Design review of the part built by this model. Coordinates are the model's own, in mm. Face numbers are marked on the shaded views. A direction names the side the tool comes from. Give positions to 0.01 mm unless a question says otherwise; leave off trailing zeros. Loops run counter-clockwise (first coordinate to the right, second up) from the corner with the lowest first, then second, coordinate; pieces in that order, holes last. Notation, with made-up numbers: (31.25, -23.75) - (73.25, -23.75) arc R24 ccw to (73.25, -5.75) - close; hole circle Ø10 at (35, -4). An arc over 180 degrees is marked (long way). One line per item, written item: value. Start each with the question number.
```python
from build123d import *

# Parameters (mm, degrees)
SKETCH1_R           = 10.5
BOSS_EXTRUDE2_DEPTH = 2
SKETCH2_W           = 40
SKETCH2_H           = 2
BOSS_EXTRUDE3_DEPTH = 35
CUT_EXTRUDE1_DEPTH  = 35
CIRPATTERN1_COUNT   = 3
SKETCH5_R           = 1.5
CUT_EXTRUDE2_DEPTH  = 35
SKETCH6_R           = 1.5
CUT_EXTRUDE3_DEPTH  = 35


with BuildPart() as part:
    # Sketch1 → Boss-Extrude2 (new body)
    with BuildSketch(Plane(origin=(0, 0, 0), x_dir=(1, 0, 0), z_dir=(0, 1, 0))):
        with BuildLine():
            Line((-18.229166667, 5.4375), (-18.229166667, -21.5625))
            Line((-18.229166667, -21.5625), (21.770833333, -21.5625))
            Line((21.770833333, -21.5625), (21.770833333, 5.4375))
            ThreePointArc((21.770833333, 5.4375), (1.770833333, 25.4375), (-18.229166667, 5.4375))
        make_face()
        with Locations(Location((1.770833333, 5.4375, 0), (0, 0, 270))):
            Circle(SKETCH1_R, mode=Mode.SUBTRACT)
    extrude(amount=BOSS_EXTRUDE2_DEPTH)

    # Sketch2 → Boss-Extrude3 (add)
    with BuildSketch(Plane(origin=(0, 2, 0), x_dir=(1, 0, 0), z_dir=(0, 1, 0))):
        with Locations((1.770833333, -20.5625)):
            Rectangle(SKETCH2_W, SKETCH2_H)
    extrude(amount=BOSS_EXTRUDE3_DEPTH)

    # Sketch4 → Cut-Extrude1 (cut)
    with BuildSketch(Plane(origin=(0, 2, 0), x_dir=(1, 0, 0), z_dir=(0, 1, 0))):
        with BuildLine():
            ThreePointArc((1.770833333, 21.4375), (0.770833333, 20.4375), (1.770833333, 19.4375))
            Line((1.770833333, 19.4375), (1.770833333, 21.4375))
        make_face()
        with BuildLine():
            Line((1.770833333, 21.4375), (1.770833333, 19.4375))
            ThreePointArc((1.770833333, 19.4375), (2.477940115, 19.730393219), (2.770833333, 20.4375))
            ThreePointArc((2.770833333, 20.4375), (2.477940115, 21.144606781), (1.770833333, 21.4375))
        make_face()
    cut_extrude1 = extrude(amount=-CUT_EXTRUDE1_DEPTH, mode=Mode.SUBTRACT)

    # CirPattern1: Cut-Extrude1 ×3 about axis
    cirpattern1_axis = Axis((1.770833333, 0, -5.4375), (0, 1, 0))
    for i in range(1, CIRPATTERN1_COUNT):
        add(cut_extrude1.rotate(cirpattern1_axis, i * 360 / CIRPATTERN1_COUNT), mode=Mode.SUBTRACT)

    # Sketch5 → Cut-Extrude2 (cut)
    with BuildSketch(Plane(origin=(0, 0, 19.5625), x_dir=(-1, 0, 0), z_dir=(0, 0, -1))):
        with Locations((-16.466888349, 10.262371912)):
            Circle(SKETCH5_R)
        with Locations((-16.470833333, 30.952470071)):
            Circle(SKETCH5_R)
    extrude(amount=-CUT_EXTRUDE2_DEPTH, mode=Mode.SUBTRACT)

    # Sketch6 → Cut-Extrude3 (cut)
    with BuildSketch(Plane(origin=(0, 0, 19.5625), x_dir=(-1, 0, 0), z_dir=(0, 0, -1))):
        with Locations((12.929166667, 30.96416702)):
            Circle(SKETCH6_R)
        with Locations((12.929166667, 10.470851603)):
            Circle(SKETCH6_R)
    extrude(amount=-CUT_EXTRUDE3_DEPTH, mode=Mode.SUBTRACT)


solid = part.part
```
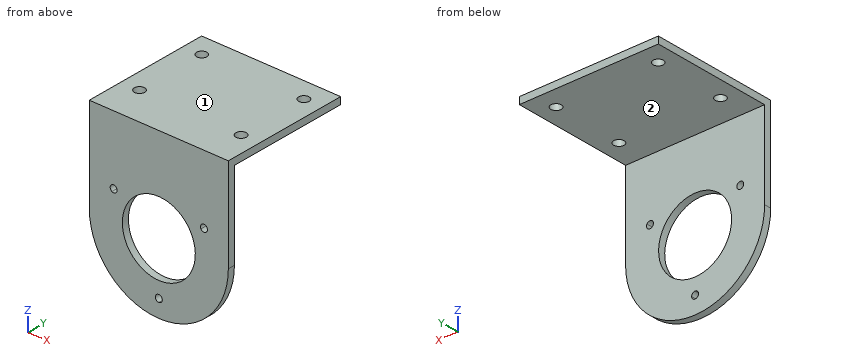
(1) Take a section at D-D on y = 19. State the section outline as (x, z) points.
(2) Take a section at B-B on z = -4. State the section outline as (x, y) points, and give its area (3 significant figures).
(3) For pin 1 Ø10.5 at (x, y) = (0, 21) entering from -Z; pin 2 Ø1.5 at (x, z) = (-11, 3.5) entering from +Y, all flat-tipped, find the tip position at first contact; note any pin that passes through.
(4) To check wall thickness, follow L1, parallel to Y at x = 1.5, z = 11.5; L2, parallel to Z at x = -3, y = 32. State the ranges of each line that lie inside material, in increasing order. Write a range as from..to.
(5) Machinability: for the marked faces 1 and 2, which of the approach directions +Z, -Z, +X, -X, +Y, -Y give a long, thin tool a straight path to every point of the face, cutting with its end or side? Answer none if there is none.
(6) Take a section at A-A on x = 7. State the section outline as (y, z) points.
(7) Take a section at C-C on z = 12. State the section outline as (x, y) points, and give its area (3 significant figures).
Here are the results:
1. outline: (-18.23, 19.56) - (21.77, 19.56) - (21.77, 21.56) - (-18.23, 21.56) - close
2. outline: (-18.23, 0) - (-8.63, 0) - (-8.63, 2) - (-18.23, 2) - close; (12.17, 0) - (21.77, 0) - (21.77, 2) - (12.17, 2) - close
2. area: 38.4 mm²
3. pin 1: z = 19.56
3. pin 2: y = 2
4. L1: 0..2
4. L2: 19.56..21.56
5. face 1: +Z, +X, -X, +Y, -Y
5. face 2: -Z, +X, -X, +Y
6. outline: (0, -24.74) - (2, -24.74) - (2, -14.54) - (0, -14.54) - close; (0, 3.67) - (2, 3.67) - (2, 19.56) - (37, 19.56) - (37, 21.56) - (0, 21.56) - close
7. outline: (-18.23, 0) - (21.77, 0) - (21.77, 2) - (-18.23, 2) - close
7. area: 80.0 mm²
